```python
from build123d import *

# Parameters (mm, degrees)
SKETCH1_R           = 34.875
SKETCH1_R_2         = 9
BOSS_EXTRUDE1_DEPTH = 6.35
SKETCH2_R           = 2
CUT_EXTRUDE1_DEPTH  = 7.35
SKETCH3_R           = 5.55625
CUT_EXTRUDE2_DEPTH  = 7.35


with BuildPart() as part:
    # Sketch1 → Boss-Extrude1 (new body)
    with BuildSketch(Plane.XY):
        Circle(SKETCH1_R)
        Circle(SKETCH1_R_2, mode=Mode.SUBTRACT)
    extrude(amount=BOSS_EXTRUDE1_DEPTH)

    # Sketch2 → Cut-Extrude1 (cut, through all)
    with BuildSketch(Plane(origin=(0, 0, 0), x_dir=(-1, 0, 0), z_dir=(0, 0, -1))):
        with Locations((-11, 11.618950039)):
            Circle(SKETCH2_R)
        with Locations((11, 11.618950039)):
            Circle(SKETCH2_R)
        with Locations((11, -11.618950039)):
            Circle(SKETCH2_R)
        with Locations((-11, -11.618950039)):
            Circle(SKETCH2_R)
    extrude(amount=-CUT_EXTRUDE1_DEPTH, mode=Mode.SUBTRACT)

    # Sketch3 → Cut-Extrude2 (cut, through all)
    with BuildSketch(Plane(origin=(0, 0, 0), x_dir=(-1, 0, 0), z_dir=(0, 0, -1))):
        with Locations((0, -27.559440888)):
            Circle(SKETCH3_R)
    extrude(amount=-CUT_EXTRUDE2_DEPTH, mode=Mode.SUBTRACT)


solid = part.part
```
Could you check a few things on this model? Use its own coordinates, in mm. Round coordinates to 2 decimals unless told otherwise and drop trailing zeros. Loops run counter-clockwise (first coordinate to the right, second up) from the corner with the lowest first, then second, coordinate; pieces in that order, holes last. Notation, with made-up numbers: M -12,78 L 5,78 A20 ccw 5,113 Z; hole C 28.5,48.5 d1. An arc over 180 degrees is marked long. Write item = value, one per line.
1. I need wall thicknesses on probe 1 along Y at (x, z) = (0, 2) (3 decimals); probe 2 along X at (y, z) = (-11, 4); probe 3 along Y at (x, z) = (2.5, 2.5). Which ranges of each line are inside material? Lowest first, please.
Results below:
probe_1 = -34.875 to -33.116, -22.003 to -9, 9 to 34.875
probe_2 = -33.09 to -12.9, -9.1 to 9.1, 12.9 to 33.09
probe_3 = -34.79 to -32.52, -22.6 to -8.65, 8.65 to 34.79
2. Thinking about a two-plate mould opening in X: for faces 1 (the face through (-27.676, -21.221, 3.131)), 2 (the face through (7, -7, 0)), 3 (the face through (1.204, -32.984, 3.131)), 4 (the face through (11.26, -9.636, 3.131)), which applies, +X half, -X half, draft (parallel to the pull), parting line (faces both ways), or undercut?
Results below:
face_1 = parting line
face_2 = draft
face_3 = undercut
face_4 = undercut
3. I want a section at B-B, the plane x = 0. Write out the boundary of the cut face in (y, z) (3 decimals), and give its area (3 significant figures).
Results below:
outline = M -34.875,0 L -33.116,0 L -33.116,6.35 L -34.875,6.35 Z; M -22.003,0 L -9,0 L -9,6.35 L -22.003,6.35 Z; M 9,0 L 34.875,0 L 34.875,6.35 L 9,6.35 Z
area = 258 mm²
4. I want a section at D-D, the plane x = 11. Write out the boundary of the cut face in (y, z), and give its area (3 significant figures).
Results below:
outline = M -33.09,0 L -13.62,0 L -13.62,6.35 L -33.09,6.35 Z; M -9.62,0 L 9.62,0 L 9.62,6.35 L -9.62,6.35 Z; M 13.62,0 L 33.09,0 L 33.09,6.35 L 13.62,6.35 Z
area = 370 mm²
5. I want a section at C-C, the plane z = 3. Count the separate pieces of the cut face and the enclosed holes in it, and give its area (3 significant figures).
Results below:
separate_pieces = 1
enclosed_holes = 6
area = 3,420 mm²
6. Will these pins go through, and if not, where does the flat tip stop? P1, Ø3, axis at x = 11, y = 11.62, coming from the -Z side; P2, Ø13, axis at x = 0, y = -27.56, coming from the -Z side; P3, Ø1.5, axis at x = 25, z = 3, coming from the +Y side; P4, Ø3, axis at x = -10, z = 2.5, coming from the -Y side.
Results below:
P1 = through
P2 = 0
P3 = 25.06
P4 = -33.82
7. I want a section at A-A, the plane y = 0. Write out the boundary of the cut face in (x, z) (3 decimals).
Results below:
outline = M -34.875,0 L -9,0 L -9,6.35 L -34.875,6.35 Z; M 9,0 L 34.875,0 L 34.875,6.35 L 9,6.35 Z
